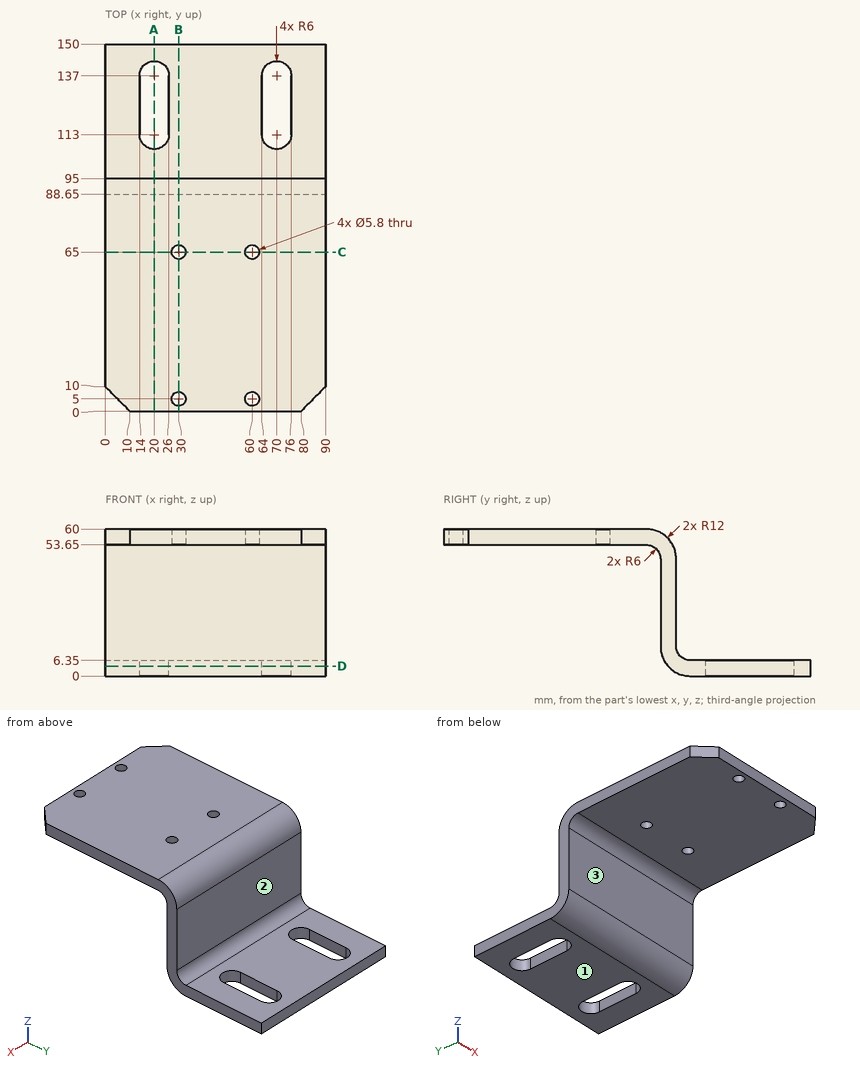
Design review of the part shown in the three views and the two pictorial views. Dimensions are in mm from the part's minimum x, y and z. A direction names the side the tool comes from. Round coordinates to 2 decimals unless told otherwise and drop trailing zeros. Write each loop counter-clockwise with the first axis right and the second up, starting at its lowest first coordinate (ties: lowest second). Pieces come first, ordered by that corner, then holes. Notation, with made-up numbers: (65.25, 43) - (114.25, 43) arc R17 cw to (114.25, 70) - close; hole circle Ø6 at (-0.5, 63.25). An arc over 180 degrees is marked (long way). Return JSON: item names as keys, results as strings. Group by question number.
Item 1: Insertion check: P1, Ø2, axis at x = 34.5, y = 104, coming from the +Z side; P2, Ø6.5, axis at x = 30, y = 5, coming from the -Z side; P3, Ø6, axis at x = 50.5, y = 87, coming from the +Z side. Each pin has a flat end and moves straight along its axis. Give the tip position at first contact, or say it passes through.
Item 2: We need section A-A on x = 20. Write out the cut boundary in (y, z).
Item 3: We need section C-C on y = 65. Write out the cut boundary in (x, z), and give its area (3 significant figures).
Item 4: We need section B-B on x = 30. Write out the cut boundary in (y, z), and give its area (3 significant figures).
Item 5: Machinability: for the marked faces 1, 2 and 3, which of the approach directions +Z, -Z, +X, -X, +Y, -Y give a long, thin tool a straight path to every point of the face, cutting with its end or side? Answer none if there is none.
Item 6: We need section D-D on z = 4. Write out the cut boundary in (x, y).
Item 7: For probe 1 along Y at (x, z) = (30, 58); probe 2 along Y at (x, z) = (30, 55.5); probe 3 along Z at (x, y) = (38.5, 107), list the stretches that pass through material, from the lowest coordinate up. Write a range as [from, to].
Model answer:
{
 "1": {"P1": "stops at z = 6.35", "P2": "stops at z = 53.65", "P3": "stops at z = 59.96"},
 "2": {"outline": "(0, 53.65) - (82.65, 53.65) arc R6 cw to (88.65, 47.65) - (88.65, 12) arc R12 ccw to (100.65, 0) - (107, 0) - (107, 6.35) - (101, 6.35) arc R6 cw to (95, 12.35) - (95, 48) arc R12 ccw to (83, 60) - (0, 60) - close; (143, 0) - (150, 0) - (150, 6.35) - (143, 6.35) - close"},
 "3": {"outline": "(0, 53.65) - (27.1, 53.65) - (27.1, 60) - (0, 60) - close; (32.9, 53.65) - (57.1, 53.65) - (57.1, 60) - (32.9, 60) - close; (62.9, 53.65) - (90, 53.65) - (90, 60) - (62.9, 60) - close", "area": "498 mm²"},
 "4": {"outline": "(0, 53.65) - (2.1, 53.65) - (2.1, 60) - (0, 60) - close; (7.9, 53.65) - (62.1, 53.65) - (62.1, 60) - (7.9, 60) - close; (67.9, 53.65) - (82.65, 53.65) arc R6 cw to (88.65, 47.65) - (88.65, 12) arc R12 ccw to (100.65, 0) - (150, 0) - (150, 6.35) - (101, 6.35) arc R6 cw to (95, 12.35) - (95, 48) arc R12 ccw to (83, 60) - (67.9, 60) - close", "area": "1,170 mm²"},
 "5": {"face 1": "-Z, +X, -X, +Y, -Y", "face 2": "+Z, +X, -X, +Y", "face 3": "-Z, +X, -X, -Y"},
 "6": {"outline": "(0, 91.71) - (90, 91.71) - (90, 150) - (0, 150) - close; hole (14, 113) arc R6 ccw to (26, 113) - (26, 137) arc R6 ccw to (14, 137) - close; hole (64, 113) arc R6 ccw to (76, 113) - (76, 137) arc R6 ccw to (64, 137) - close"},
 "7": {"probe 1": "y = [0, 2.1], [7.9, 62.1], [67.9, 89.63]", "probe 2": "y = [0, 2.1], [7.9, 62.1], [67.9, 92.37]", "probe 3": "z = [0, 6.35]"}
}
